Part model, mm, in its own coordinate system. Coordinates: 2 decimals unless noted, no trailing zeros. Loops run counter-clockwise (first coordinate to the right, second up) from the corner with the lowest first, then second, coordinate; pieces in that order, holes last.
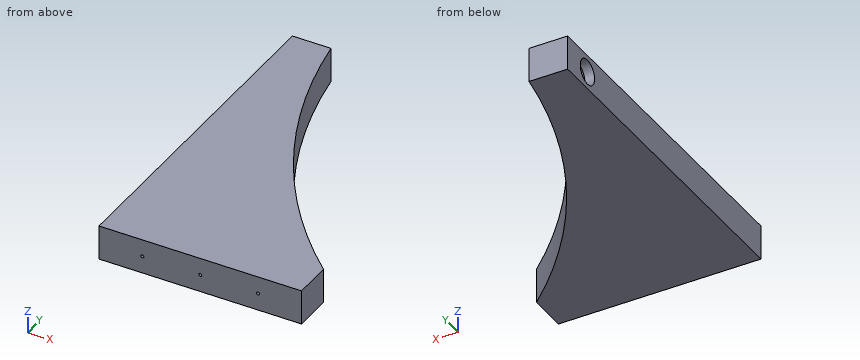
Autodesk Inventor part; units mm, degrees
ref_plane "YZ Plane" through (0, 0, 0) normal (1, 0, 0) x (0, 1, 0)
ref_plane "XZ Plane" through (0, 0, 0) normal (0, 1, 0) x (-1, 0, 0)
ref_plane "XY Plane" through (0, 0, 0) normal (0, 0, 1) x (1, 0, 0)
sketch "Sketch1" plane through (0, 0, 0) normal (0, 0, 1) x (1, 0, 0)
  line L0 (0, 0) -> (140, 0) construction
  line L1 (140, 0) -> (140, 300) construction
  line L2 (140, 300) -> (0, 300) construction
  line L3 (0, 300) -> (0, 0) construction
  line L4 (70, 308.6686) -> (70, 317.1965) construction
  line L5 (130, 290) -> (130, 293.3347) construction
  line L6 (0, 160.5) -> (-18, 160.5) construction
  line L7 (-18, 160.5) -> (-18, 180.5) construction
  line L8 (-18, 180.5) -> (0, 180.5) construction
  line L9 (0, 180.5) -> (0, 160.5) construction
  line L10 (-16.3067, 150) -> (-26.4998, 150) construction
  circle A0 centre (-9, 170.5) radius 3 construction
  line L11 (-18, 180.5) -> (0, 200.5) construction
  line L12 (0, 139.5) -> (-18, 139.5) construction
  line L13 (-18, 139.5) -> (-18, 119.5) construction
  circle A1 centre (-9, 129.5) radius 3 construction
  line L14 (-18, 119.5) -> (0, 99.5) construction
  line L15 (140, 160.5) -> (158, 160.5) construction
  line L16 (158, 160.5) -> (158, 180.5) construction
  circle A2 centre (149, 170.5) radius 3 construction
  line L17 (158, 180.5) -> (140, 200.5) construction
  line L18 (158, 139.5) -> (158, 119.5) construction
  line L19 (140, 139.5) -> (158, 139.5) construction
  circle A3 centre (149, 129.5) radius 3 construction
  line L20 (158, 119.5) -> (140, 99.5) construction
  line L21 (158, 186) -> (140, 186) construction
  line L22 (140, 186) -> (140, 114) construction
  line L23 (140, 114) -> (158, 114) construction
  line L24 (158, 114) -> (158, 186) construction
  line L25 (158, 156.5) -> (153, 156.5) construction
  line L26 (153, 156.5) -> (153, 143.5) construction
  line L27 (153, 143.5) -> (158, 143.5) construction
  line L28 (158, 143.5) -> (158, 156.5) construction
  line L29 (153, 152) -> (165, 152) construction
  line L30 (165, 152) -> (165, 148) construction
  line L31 (165, 148) -> (153, 148) construction
  line L32 (153, 148) -> (153, 152) construction
  line L33 (158.25, 155.5) -> (159.85, 155.5) construction
  line L34 (159.85, 155.5) -> (159.85, 144.5) construction
  line L35 (159.85, 144.5) -> (158.25, 144.5) construction
  line L36 (158.25, 144.5) -> (158.25, 155.5) construction
  line L37 (160.1, 156.5) -> (165.1, 156.5) construction
  line L38 (165.1, 156.5) -> (165.1, 143.5) construction
  line L39 (165.1, 143.5) -> (160.1, 143.5) construction
  line L40 (160.1, 143.5) -> (160.1, 156.5) construction
  line L41 (160.1, 166.5) -> (160.1, -9)
  line L42 (160.1, 166.5) -> (180.1, 166.5)
  line L43 (160.1, -9) -> (70, -9) construction
  line L44 (160.1, -9) -> (265.1, -9)
  line L45 (265.1, -9) -> (265.1, 11)
  arc A4 (180.1, 166.5) -> (265.1, 11) centre (442.3295, 208.8594) ccw
  point P0 (70, 300)
  point P1 (10, 150)
  point P2 (0, 150)
  point P3 (70, 312.9325)
  point P4 (-21.4032, 150)
  point P5 (-18, 170.5)
  point P6 (-9, 180.5)
  point P7 (153, 150)
  point P8 (140, 150)
  point P9 (153, 150)
  point P10 (158.25, 150)
  dimension "d0" = 140
  dimension "d1" = 300
  dimension "d85" = 18
  dimension "d86" = 20
  dimension "d87" = 10.5
  dimension "d88" = 6
  dimension "d89" = 20
  dimension "racewidth" = 5
  dimension "d110" = 13
  dimension "d111" = 12
  dimension "d112" = 4
  dimension "d113" = 1.6
  dimension "d114" = 5
  dimension "d117" = 11
  dimension "gap" = 0.25
  dimension "d119" = 0.25
  dimension "d120" = 0
  dimension "d121" = 10
  dimension "d122" = 20
  dimension "d123" = 9
  dimension "d124" = 20.1
  dimension "d126" = 105
  dimension "d127" = 20
  dimension "d128" = 0.1
  dimension "d129" = 175.5
  dimension "d132" = 16.5
  dimension "d147" = 90.1
  dimension "d148" = 2.1
extrude "Extrusion1" add sketch "Sketch1" along normal blind 18
sketch "Sketch2" plane through (160.1, -9, 0) normal (-1, 0, 0) x (0, 0, 1)
  circle A0 centre (9, 157.5) radius 6.5
  line L0 (0, 175.5) -> (18, 175.5)
  point P0 (0, 9)
  point P1 (9, 175.5)
  dimension "bearingdiameter" = 13
  dimension "d134" = 18
extrude "Extrusion2" cut sketch "Sketch2" against normal blind 5
sketch "Sketch3" plane through (160.1, -9, 0) normal (0, -1, 0) x (1, 0, 0)
  circle A0 centre (22.5, 9) radius 0.75
  line L0 (0, 0) -> (0, 18)
  line L1 (0, 0) -> (105, 0)
  circle A1 centre (52.5, 9) radius 0.75
  circle A2 centre (82.5, 9) radius 0.75
  point P0 (-160.1, 0)
  point P1 (0, 9)
  point P2 (52.5, 0)
  dimension "d137" = 1.5
  dimension "d140" = 30
extrude "Extrusion3" cut sketch "Sketch3" against normal blind 22
properties part number "arms"
Q1. Saw through at A-A (z = 12.25). List the corners of the cut face in (x, y).
Q2. Saw through at B-B (y = 148.5). List the corners of the cut face in (x, z).
Q3. Saw through at D-D (y = 77). List the corners of the cut face in (x, z), plus the area to 3 significant figures.
Q4. Saw through at C-C (x = 222). List the corners of the cut face in (y, z).
Q5. Drop flat-ended pins along their axis: P1, Ø1.4, axis at x = 242.6, z = 9, coming from the +Y side; P2, Ø1.7, axis at x = 212.6, z = 9, coming from the +Y side; P3, Ø8, axis at x = 239, z = 8, coming from the +Y side. Give the stop position or say it passes through.
Q6. Probe line 1 (Z direction, x = 242.6, y = -4.5); line 2 (Y direction, x = 164, z = 9); line 3 (X direction, y = 4.5, z = 8.5). List the from-to ranges inside material, lowest first.
Checked values:
1. outline: (160.1, -9) - (265.1, -9) - (265.1, 11) arc R265.63 cw to (180.1, 166.5) - (160.1, 166.5) - (160.1, 154.13) - (165.1, 154.13) - (165.1, 142.87) - (160.1, 142.87) - close
2. outline: (160.1, 0) - (183.65, 0) - (183.65, 18) - (160.1, 18) - (160.1, 15.5) - (165.1, 15.5) - (165.1, 2.5) - (160.1, 2.5) - close
3. outline: (160.1, 0) - (211.74, 0) - (211.74, 18) - (160.1, 18) - close
3. area: 930 mm2
4. outline: (-9, 0) - (60.49, 0) - (60.49, 18) - (-9, 18) - close
5. P1: stops at y = 34.54
5. P2: stops at y = 76.98
5. P3: stops at y = 42.81
6. line 1: z = 0 to 8.25, 9.75 to 18
6. line 2: y = -9 to 142, 155 to 166.5
6. line 3: x = 160.1 to 182.04, 183.16 to 212.04, 213.16 to 242.04, 243.16 to 265.1
